from build123d import *

# Parameters (mm, degrees)
F0_R           = 1.75
F0_R_2         = 1.5
F1_DEPTH       = 18
F2_SIZE        = 5
F3_R           = 8
F4_D           = 7.2
F4_DEPTH       = 35
F4_CBORE_D     = 11
F4_CBORE_DEPTH = 6
F4_TIP         = 2.1630982285


# Not quite as in the source:
# - a feature names something its author has since deleted; it is built from what else it names


with BuildPart() as f1:
    # F0 (on Front) → F1 (new body)
    with BuildSketch(Plane.XZ):
        with BuildLine():
            ThreePointArc((-18.125, 0), (0, 18.125), (18.125, 0))
            Line((18.125, 0), (31.75, 0))
            Line((31.75, 0), (31.75, 31.75))
            Line((31.75, 31.75), (-31.75, 31.75))
            Line((-31.75, 31.75), (-31.75, 0))
            Line((-31.75, 0), (-18.125, 0))
        make_face()
        with Locations((-23.6880771697, 23.6880771697)):
            Circle(F0_R, mode=Mode.SUBTRACT)
        with Locations((-15.5563491861, 15.5563491861)):
            Circle(F0_R, mode=Mode.SUBTRACT)
        with Locations((15.5563491861, 15.5563491861)):
            Circle(F0_R, mode=Mode.SUBTRACT)
        with Locations((23.6880771697, 23.6880771697)):
            Circle(F0_R, mode=Mode.SUBTRACT)
        with BuildLine():
            Line((31.75, 0), (18.125, 0))
            ThreePointArc((18.125, 0), (0, -18.125), (-18.125, 0))
            Line((-18.125, 0), (-31.75, 0))
            Line((-31.75, 0), (-31.75, -31.75))
            Line((-31.75, -31.75), (31.75, -31.75))
            Line((31.75, -31.75), (31.75, 0))
        make_face()
        with Locations((-23.6880771697, -23.6880771697)):
            Circle(F0_R, mode=Mode.SUBTRACT)
        with Locations((-15.5563491861, -15.5563491861)):
            Circle(F0_R, mode=Mode.SUBTRACT)
        with Locations((23.6880771697, -23.6880771697)):
            Circle(F0_R, mode=Mode.SUBTRACT)
        with Locations((15.5563491861, -15.5563491861)):
            Circle(F0_R, mode=Mode.SUBTRACT)
        Polygon((57.25, 0), (31.75, 0), (31.75, -31.75), (-31.75, -31.75), (-31.75, 0), (-49.75, 0), (-49.75, -46), (57.25, -46), align=None)
        with Locations((-42, -31)):
            Circle(F0_R_2, mode=Mode.SUBTRACT)
        with Locations((49.5, -31)):
            Circle(F0_R_2, mode=Mode.SUBTRACT)
    extrude(amount=F1_DEPTH)

    # F2
    f2_edges = [f1.edges().sort_by_distance(p)[0] for p in [
        (-49.75, -9, -46),
        (57.25, -9, -46),
    ]]
    chamfer(f2_edges, length=F2_SIZE)

    # F3
    f3_edges = [f1.edges().sort_by_distance(p)[0] for p in [
        (-31.75, -9, 0),
        (-31.75, -9, 31.75),
        (31.75, -9, 31.75),
        (31.75, -9, 0),
    ]]
    fillet(f3_edges, radius=F3_R)

    # F4
    with Locations(Plane(origin=(0, 0, 0), x_dir=(1, 0, 0), z_dir=(0, 1, 0))):
        with Locations((49.5, 18), (-42, 18)):
            CounterBoreHole(F4_D / 2, F4_CBORE_D / 2, F4_CBORE_DEPTH, depth=F4_DEPTH)
            with Locations((0, 0, -(F4_DEPTH + F4_TIP / 2))):  # 118° drill point
                Cone(0, F4_D / 2, F4_TIP, mode=Mode.SUBTRACT)


solid = f1.part
Verification items for the finished model (mm, model axes). A direction names the side the tool comes from. Coordinates: 2 decimals unless noted, no trailing zeros. Loops run counter-clockwise (first coordinate to the right, second up) from the corner with the lowest first, then second, coordinate; pieces in that order, holes last. Notation, with made-up numbers: (77, -14.5) -> (81, -14.5) arc R27 cw to (81, 9.5) -> close; hole circle Ø10 at (34.25, -29.5). An arc over 180 degrees is marked (long way). Answer as a JSON object with one key per item and string values. Group by question number.
Item 1: Sectioned sample at D-D on z = -10. Record the boundary of the cut face in (x, y).
Item 2: Depth check by flat-ended pin: pin 1 (5.5 mm diameter, centred on x = 15.56, z = -15.56, fed in from -Y); pin 2 (5 mm diameter, centred on x = -46.5, y = -11, fed in from +Z); pin 3 (1 mm diameter, centred on y = -9, z = 15, fed in from -X); pin 4 (3 mm diameter, centred on x = -23.69, z = 23.69, fed in from +Y). Enter the tip coordinate at first touch or a pass-through.
Item 3: Sectioned sample at A-A on z = -31. Record the boundary of the cut face in (x, y).
Item 4: Sectioned sample at C-C on x = -42. Record the boundary of the cut face in (y, z).
Item 5: Sectioned sample at B-B on x = 0. Record the boundary of the cut face in (y, z) (3 decimals), plus the area to 3 significant figures.
Item 6: Tool access check on faces 1 (the flat face through (31.75, -9, 16)), 2 (the flat face through (-31.75, -9, 16)), 3 (the flat face through (-38, -6, -17)). Record the directions out of +Z, -Z, +X, -X, +Y, -Y that give a thin tool (end or side, any length) a straight path to the whole face; none if there is none.
Item 7: Scan lines: probe 1 along X at (y, z) = (-2.5, 23.5); probe 2 along Z at (x, y) = (-42, -9.5); probe 3 along Z at (x, y) = (0, -5) (3 decimals). Record each from-to range of solid material in increasing order.
Item 8: Mould release check, pull along Z, two halves, no side actions. Record for faces 4 (the cylindrical face through (44, -3, -18)), 5 (the flat face through (3, -9, -46)), 6 (the flat face through (-49.75, -9, -20)): +Z half, -Z half, draft (parallel to the pull), parting line (faces both ways), or undercut.
Evaluation:
{
 "1": {"outline": "(-49.75, -18) -> (-15.12, -18) -> (-15.12, 0) -> (-49.75, 0) -> close; (15.12, -18) -> (57.25, -18) -> (57.25, 0) -> (15.12, 0) -> close"},
 "2": {"pin 1": "stops at y = -18", "pin 2": "stops at z = 0", "pin 3": "stops at x = -31.75", "pin 4": "passes through"},
 "3": {"outline": "(-49.75, -18) -> (-43.5, -18) -> (-43.5, 0) -> (-49.75, 0) -> close; (-40.5, -18) -> (48, -18) -> (48, 0) -> (-40.5, 0) -> close; (51, -18) -> (57.25, -18) -> (57.25, 0) -> (51, 0) -> close"},
 "4": {"outline": "(-18, -46) -> (0, -46) -> (0, -32.5) -> (-18, -32.5) -> close; (-18, -29.5) -> (0, -29.5) -> (0, -23.5) -> (-6, -23.5) -> (-6, -21.6) -> (-18, -21.6) -> close; (-18, -14.4) -> (-6, -14.4) -> (-6, -12.5) -> (0, -12.5) -> (0, 0) -> (-18, 0) -> close"},
 "5": {"outline": "(-18, -46) -> (0, -46) -> (0, -18.125) -> (-18, -18.125) -> close; (-18, 18.125) -> (0, 18.125) -> (0, 31.75) -> (-18, 31.75) -> close", "area": "747 mm²"},
 "6": {"face 1": "+Z, +X, +Y, -Y", "face 2": "+Z, -X, +Y, -Y", "face 3": "+Y"},
 "7": {"probe 1": "x = -31.75 to -25.43, -21.95 to 21.95, 25.43 to 31.75", "probe 2": "z = -46 to -32.5, -29.5 to -21.6, -14.4 to 0", "probe 3": "z = -46 to -18.125, 18.125 to 31.75"},
 "8": {"face 4": "undercut", "face 5": "-Z half", "face 6": "draft"}
}
